Input: part model. Units: mm. Frame: model coordinates. Face numbers are marked on the shaded views. A direction names the side the tool comes from. Round coordinates to 2 decimals unless told otherwise and drop trailing zeros. Order: outer loops, then holes, each group sorted by start corner. A loop starts at its lowest first (then second) coordinate and runs counter-clockwise, first axis right, second up.
Item 1: Reachability of the marked faces 1, 2 and 3 from +Z, -Z, +X, -X, +Y, -Y: full face, straight path, thin tool, end or side. Return the list, or none.
Item 2: Cut plane C-C on y = 0. Output: boundary loops of the cut face in (x, z).
Item 3: Cut plane B-B on x = 16.5. Output: boundary loops of the cut face in (y, z).
Item 4: Cut plane A-A on z = 7. Output: boundary loops of the cut face in (x, y), then the cut area to 3 significant figures.
Item 5: First-contact query: pin 1 (22.5 mm diameter, centred on x = -19.5, y = 0.5, fed in from +Z); pin 2 (12 mm diameter, centred on x = 5.5, y = -39.5, fed in from +Z); pin 3 (8 mm diameter, centred on x = -9.5, z = 15.5, fed in from +Y). Flat tips, straight axial feed; report the tip coordinate or a pass-through.
Item 6: Line query: L1, parallel to Y at x = -5.5, z = 1.5; L2, parallel to Y at x = 15, z = 9; L3, parallel to Z at x = 23, y = -41.5. Output: solid intervals per line, ascending.
Item 7: Cut plane D-D on z = 18. Output: boundary loops of the cut face in (x, y).
```python
from build123d import *

# Parameters (mm, degrees)
F3_DEPTH  = 10
F4_W      = 80
F4_H      = 10
F5_DEPTH  = 10
F6_R      = 5
F8_DEPTH  = 10
F10_DEPTH = 5
F12_DEPTH = 10


with BuildPart() as f3:
    # F2 (on Top) → F3 (new body)
    with BuildSketch(Plane.XY):
        with BuildLine():
            Line((35, 50), (-35, 50))
            ThreePointArc((-35, 50), (-38.5355339059, 48.5355339059), (-40, 45))
            Line((-40, 45), (-40, -45))
            ThreePointArc((-40, -45), (-38.5355339059, -48.5355339059), (-35, -50))
            Line((-35, -50), (35, -50))
            ThreePointArc((35, -50), (38.5355339059, -48.5355339059), (40, -45))
            Line((40, -45), (40, 45))
            ThreePointArc((40, 45), (38.5355339059, 48.5355339059), (35, 50))
        make_face()
    extrude(amount=F3_DEPTH)

    # F4 (on face) → F5 (join)
    with BuildSketch(Plane.XY.offset(10)):
        with Locations((0, -30)):
            Rectangle(F4_W, F4_H)
    extrude(amount=F5_DEPTH)

    # F6
    f6_edges = [f3.edges().sort_by_distance(p)[0] for p in [
        (40, -30, 20),
        (-40, -30, 20),
    ]]
    fillet(f6_edges, radius=F6_R)

    # F7 (on face) → F8 (cut, through all)
    with BuildSketch(Plane.XY.offset(10)):
        with BuildLine():
            Line((27.587, 27.413), (-27.587, 27.413))
            ThreePointArc((-27.587, 27.413), (-29.293248663, 26.706248663), (-30, 25))
            ThreePointArc((-30, 25), (-29.293248663, 23.293751337), (-27.587, 22.587))
            Line((-27.587, 22.587), (27.587, 22.587))
            ThreePointArc((27.587, 22.587), (29.293248663, 23.293751337), (30, 25))
            ThreePointArc((30, 25), (29.293248663, 26.706248663), (27.587, 27.413))
        make_face()
    extrude(amount=-F8_DEPTH, mode=Mode.SUBTRACT)

    # F9 (on face) → F10 (cut)
    with BuildSketch(Plane.XY.offset(10)):
        with BuildLine():
            Line((30, 29.7371), (-30, 29.7371))
            ThreePointArc((-30, 29.7371), (-34.7371, 25), (-30, 20.2629))
            Line((-30, 20.2629), (30, 20.2629))
            ThreePointArc((30, 20.2629), (34.7371, 25), (30, 29.7371))
        make_face()
    extrude(amount=-F10_DEPTH, mode=Mode.SUBTRACT)

    # F11 (on face) → F12 (cut, through all)
    with BuildSketch(Plane.XY.offset(10)):
        with BuildLine():
            ThreePointArc((-40, -2.5), (-37.5, 0), (-40, 2.5))
            Line((-40, 2.5), (-40, -2.5))
        make_face()
        with BuildLine():
            Line((40, -2.5), (40, 2.5))
            ThreePointArc((40, 2.5), (37.5, 0), (40, -2.5))
        make_face()
    extrude(amount=-F12_DEPTH, mode=Mode.SUBTRACT)


solid = f3.part
```
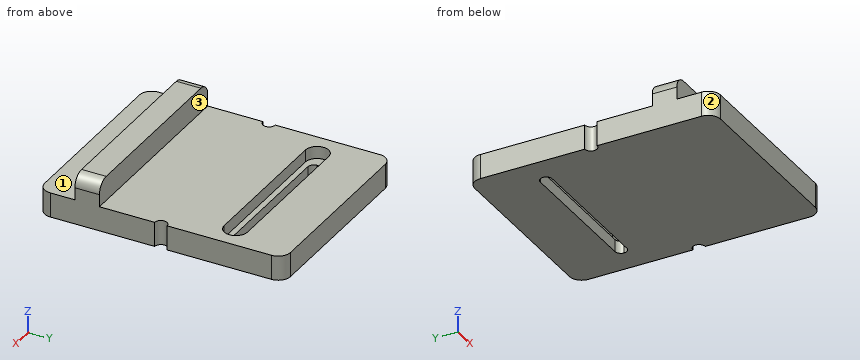
From the geometry:
1. face 1: +Z, +X, -X, -Y
1. face 2: +Z, -Z, -X, -Y
1. face 3: +Z, +X, -X, +Y
2. outline: (-37.5, 0) - (37.5, 0) - (37.5, 10) - (-37.5, 10) - close
3. outline: (-50, 0) - (22.59, 0) - (22.59, 5) - (20.26, 5) - (20.26, 10) - (-25, 10) - (-25, 20) - (-35, 20) - (-35, 10) - (-50, 10) - close; (27.41, 0) - (50, 0) - (50, 10) - (29.74, 10) - (29.74, 5) - (27.41, 5) - close
4. outline: (-40, -45) arc R5 ccw to (-35, -50) - (35, -50) arc R5 ccw to (40, -45) - (40, -2.5) arc R2.5 cw to (40, 2.5) - (40, 45) arc R5 ccw to (35, 50) - (-35, 50) arc R5 ccw to (-40, 45) - (-40, 2.5) arc R2.5 cw to (-40, -2.5) - close; hole (-30, 20.26) - (30, 20.26) arc R4.74 ccw to (30, 29.74) - (-30, 29.74) arc R4.74 ccw to start
4. area: 7,320 mm2
5. pin 1: stops at z = 10
5. pin 2: stops at z = 20
5. pin 3: stops at y = -25
6. L1: y = -50 to 22.59, 27.41 to 50
6. L2: y = -50 to 20.26, 29.74 to 50
6. L3: z = 0 to 10
7. outline: (-39, -35) - (39, -35) - (39, -25) - (-39, -25) - close
